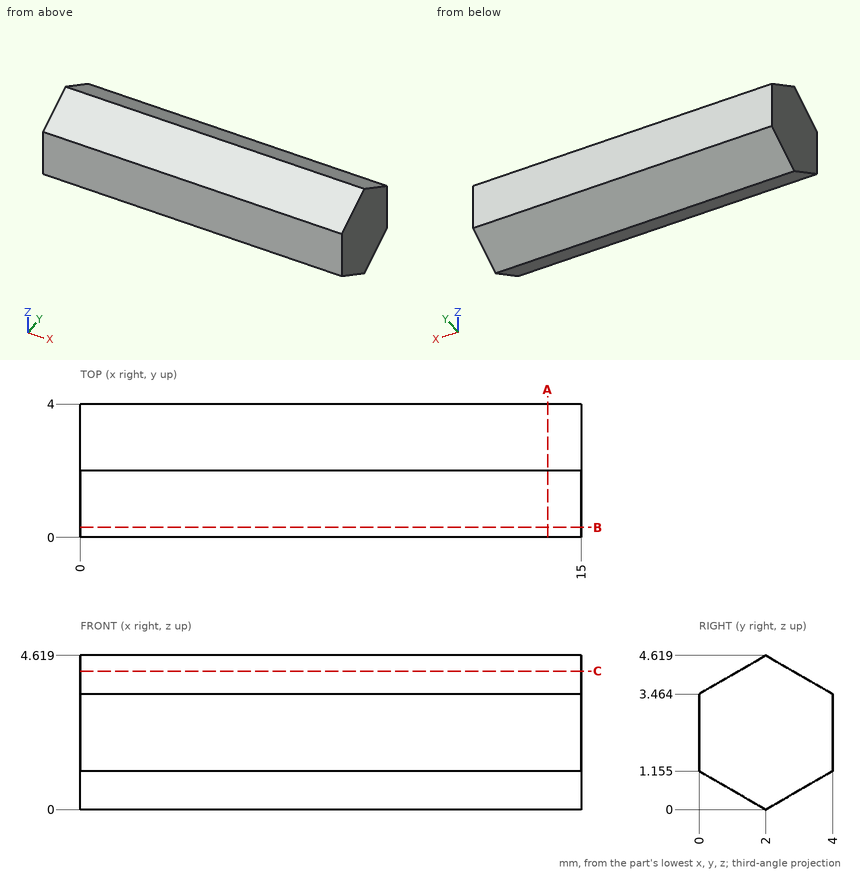
Verification items for this drawing (mm, ordinates from the low corner). Round coordinates to 2 decimals unless told otherwise and drop trailing zeros. Order: outer loops, then holes, each group sorted by start corner. A loop starts at its lowest first (then second) coordinate and runs counter-clockwise, first axis right, second up. Notation, with made-up numbers: M 1.25,36.25 L 35.25,36.25 A23 ccw 35.25,73.25 Z; hole C 86.5,51.5 d9. An arc over 180 degrees is marked long. Answer in a Markdown table with one row per item. Add a question column.
Item 1: Sectioned sample at B-B, the plane y = 0.3. Enter the section's corners in (x, z).
Item 2: Sectioned sample at C-C, the plane z = 4.15. Enter the section's corners in (x, y).
Item 3: Depth check by flat-ended pin: pin 1 Ø2 at (x, y) = (11.5, 3.5) entering from +Z. Enter the tip coordinate at first touch or a pass-through.
Item 4: Material ranges on L1, parallel to Z at x = 6, y = 3.75; L2, parallel to Z at x = 6.5, y = 2.95; L3, parallel to Y at x = 1.5, z = 0.5 (1 decimal), recorded low to high. Write a range as [from, to].
Item 5: Sectioned sample at A-A, the plane x = 14. Enter the section's corners in (y, z) (1 decimal).
Filled in:
| question | item | result |
|---|---|---|
| 1 | outline | M 0,0.98 L 15,0.98 L 15,3.64 L 0,3.64 Z |
| 2 | outline | M 0,1.19 L 15,1.19 L 15,2.81 L 0,2.81 Z |
| 3 | pin 1 | stops at z = 4.33 |
| 4 | L1 | z = [1.01, 3.61] |
| 4 | L2 | z = [0.55, 4.07] |
| 4 | L3 | y = [1.1, 2.9] |
| 5 | outline | M 0,1.2 L 2,0 L 4,1.2 L 4,3.5 L 2,4.6 L 0,3.5 Z |
